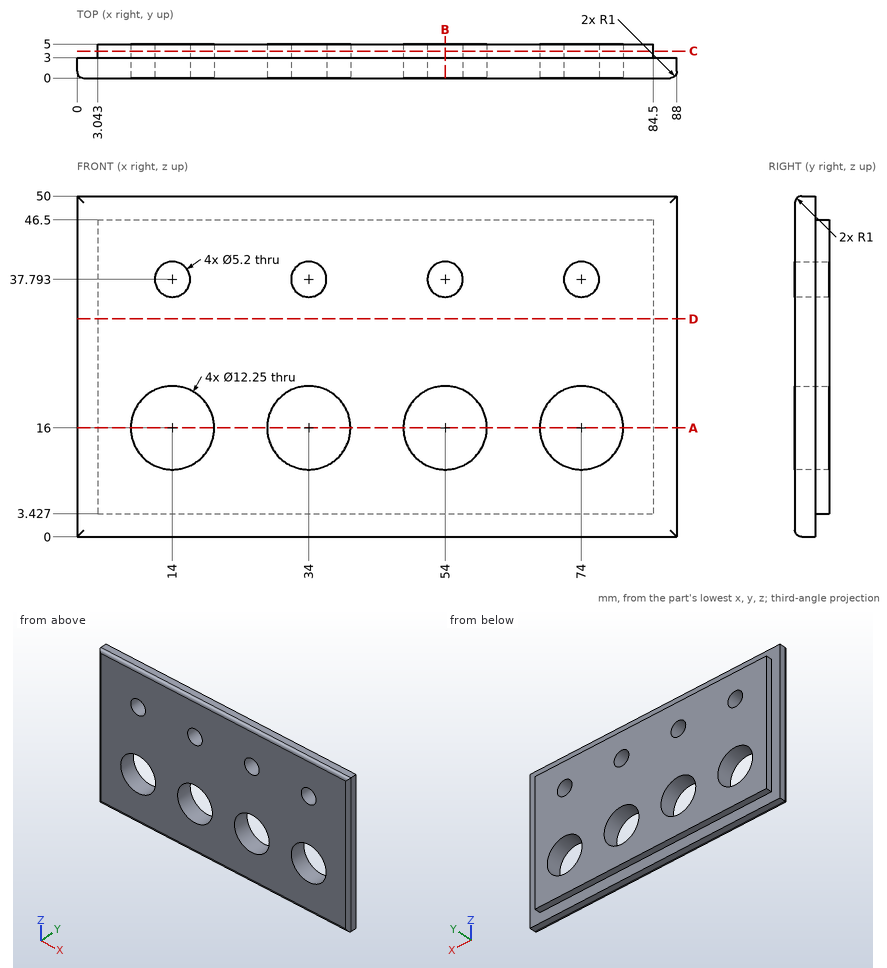
Source: three-view drawing plus pictorial views. Frame: mm from the lowest corner of the part. Round coordinates to 2 decimals unless told otherwise and drop trailing zeros. Write each loop counter-clockwise with the first axis right and the second up, starting at its lowest first coordinate (ties: lowest second). Pieces come first, ordered by that corner, then holes. Notation, with made-up numbers: M -11,-1.75 L 11,-1.75 A9 ccw 11,5.25 Z; hole C -39,3 d3. An arc over 180 degrees is marked long. Write item = value, one per line.
Item 1: Material intervals for line 1 along X through (y, z) = (1.5, 16) (1 decimal); line 2 along Z through (x, y) = (74, 2.6) (1 decimal); line 3 along Z through (x, y) = (54, 3.7) (1 decimal), sorted ascending. Write a range as [from, to].
Findings:
line_1 = [0, 7.9], [20.1, 27.9], [40.1, 47.9], [60.1, 67.9], [80.1, 88]
line_2 = [0, 9.9], [22.1, 35.2], [40.4, 50]
line_3 = [3.4, 9.9], [22.1, 35.2], [40.4, 46.5]
Item 2: Section query A-A on z = 16. Return loops of the section in (x, y) (1 decimal).
Findings:
outline = M 0,1 A1 ccw 1,0 L 7.9,0 L 7.9,5 L 3,5 L 3,3 L 0,3 Z; M 20.1,0 L 27.9,0 L 27.9,5 L 20.1,5 Z; M 40.1,0 L 47.9,0 L 47.9,5 L 40.1,5 Z; M 60.1,0 L 67.9,0 L 67.9,5 L 60.1,5 Z; M 80.1,0 L 87,0 A1 ccw 88,1 L 88,3 L 84.5,3 L 84.5,5 L 80.1,5 Z
Item 3: Section query B-B on x = 54. Return loops of the section in (y, z) (1 decimal).
Findings:
outline = M 0,1 A1 ccw 1,0 L 3,0 L 3,3.4 L 5,3.4 L 5,9.9 L 0,9.9 Z; M 0,22.1 L 5,22.1 L 5,35.2 L 0,35.2 Z; M 0,40.4 L 5,40.4 L 5,46.5 L 3,46.5 L 3,50 L 1,50 A1 ccw 0,49 Z
Item 4: Section query C-C on y = 3.95. State how many separate pieces and enclosed holes the cut face has, then the cut area to 3 significant figures.
Findings:
separate_pieces = 1
enclosed_holes = 8
area = 2,950 mm^2
Item 5: Pin query (flat end, axial travel): P1, Ø10, axis at x = 14, z = 16, coming from the -Y side (3 decimals); P2, Ø1, axis at y = 4, z = 27, coming from the +X side; P3, Ø0.6, axis at y = 4.5, z = 27.5, coming from the -X side. Return the tip coordinate at first contact, or that it passes through.
Findings:
P1 = through
P2 = 84.5
P3 = 3.04
Item 6: Section query D-D on z = 32. Return loops of the section in (x, y).
Findings:
outline = M 0,1 A1 ccw 1,0 L 87,0 A1 ccw 88,1 L 88,3 L 84.5,3 L 84.5,5 L 3.04,5 L 3.04,3 L 0,3 Z
